```python
from build123d import *

# Parameters (mm, degrees)
BOSS_EXTRUDE1_DEPTH = 2.54
SKETCH2_R           = 2.032
CUT_EXTRUDE1_DEPTH  = 61.316926471


with BuildPart() as part:
    # Sketch1 → Boss-Extrude1 (new body)
    with BuildSketch(Plane.XY):
        with BuildLine():
            Line((-18.135713172, 23.369697581), (-2.946569758, 22.862546371))
            ThreePointArc((-2.946569758, 22.862546371), (1.365281203, 25.533694473), (0.557997895, 30.541227253))
            ThreePointArc((0.557997895, 30.541227253), (-21.942363625, 40.125896641), (-44.092394737, 29.757276792))
            ThreePointArc((-44.092394737, 29.757276792), (-43.193963557, 24.360517848), (-38.053791843, 26.234236193))
            ThreePointArc((-38.053791843, 26.234236193), (-37.941623484, 26.499357867), (-37.800175961, 26.750084494))
            ThreePointArc((-37.800175961, 26.750084494), (-33.769573387, 30.919616017), (-28.44204105, 33.2105))
            ThreePointArc((-28.44204105, 33.2105), (-21.549726751, 32.845355593), (-17.268032218, 27.432))
            Line((-17.268032218, 27.432), (-21.082, 26.416))
            ThreePointArc((-21.082, 26.416), (-20.2249274, 24.29700469), (-18.135713172, 23.369697581))
        make_face()
    extrude(amount=BOSS_EXTRUDE1_DEPTH)

    # Sketch2 → Cut-Extrude1 (cut, through all)
    with BuildSketch(Plane.XY.offset(2.54)):
        with Locations((-2.794, 27.432)):
            Circle(SKETCH2_R)
    extrude(amount=-CUT_EXTRUDE1_DEPTH, mode=Mode.SUBTRACT)


solid = part.part
```
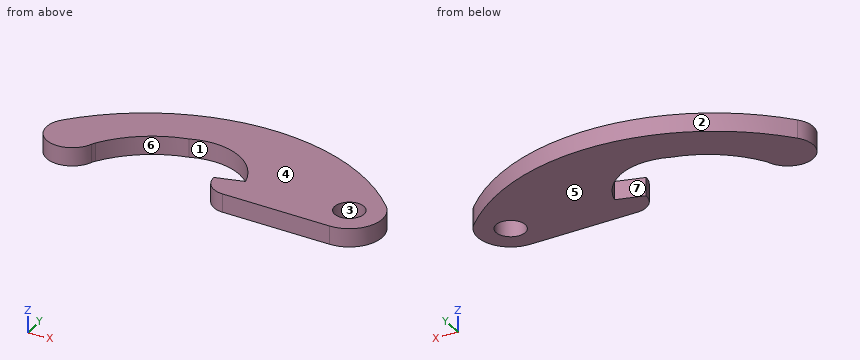
Geometry: final body of the model. Coordinates: model frame, mm. Face numbers are marked on the shaded views. A direction names the side the tool comes from. Give positions to 0.01 mm unless a question says otherwise; leave off trailing zeros. Loops run counter-clockwise (first coordinate to the right, second up) from the corner with the lowest first, then second, coordinate; pieces in that order, holes last. Notation, with made-up numbers: (59.25, 89.25) -> (63.25, 89.25) arc R10 ccw to (63.25, 99.25) -> close; hole circle Ø3 at (87, 64). An arc over 180 degrees is marked (long way). Use one line per item in the form item = value.
Item 1: Section query C-C on x = -26. Output: boundary loops of the cut face in (y, z), and give its area (3 significant figures).
A:
outline = (33.76, 0) -> (39.78, 0) -> (39.78, 2.54) -> (33.76, 2.54) -> close
area = 15.3 mm^2
Item 2: Draft query along X for the marked faces 1, 2, 3 and 4. Return one class per face: pulls with the +X half, pulls with the -X half, needs draft (parallel to the pull), parting line crosses it, or undercut.
A:
face_1 = undercut
face_2 = parting line crosses it
face_3 = undercut
face_4 = needs draft
Item 3: Section query A-A on z = 1.2. Output: boundary loops of the cut face in (x, y), and give its area (3 significant figures).
A:
outline = (-44.09, 29.76) arc R3.56 ccw (long way) to (-38.05, 26.23) arc R2.54 cw to (-37.8, 26.75) arc R14.73 cw to (-28.44, 33.21) arc R8.38 cw to (-17.27, 27.43) -> (-21.08, 26.42) arc R3.05 ccw to (-18.14, 23.37) -> (-2.95, 22.86) arc R4.57 ccw to (0.56, 30.54) arc R29.97 ccw to start; hole circle Ø4.06 at (-2.79, 27.43)
area = 442 mm^2
Item 4: Section query B-B on y = 28.5. Output: boundary loops of the cut face in (x, z), and give its area (3 significant figures).
A:
outline = (-44.79, 0) -> (-36.48, 0) -> (-36.48, 2.54) -> (-44.79, 2.54) -> close; (-17.61, 0) -> (-4.52, 0) -> (-4.52, 2.54) -> (-17.61, 2.54) -> close; (-1.07, 0) -> (1.65, 0) -> (1.65, 2.54) -> (-1.07, 2.54) -> close
area = 61.3 mm^2
Item 5: Section query D-D on y = 38.5. Output: boundary loops of the cut face in (x, z).
A:
outline = (-31.17, 0) -> (-11.67, 0) -> (-11.67, 2.54) -> (-31.17, 2.54) -> close
Item 6: Access query for the marked faces 5, 6 and 7. Directions: +Z, -Z, +X, -X, +Y, -Y. A direction counts if a zero-diameter tool reaches every point of the face in a straight line with its end or side. Return the directions, or none.
A:
face_5 = -Z, +X, -X, +Y, -Y
face_6 = +Z, -Z, -Y
face_7 = +Z, -Z
Item 7: Line query: probe 1 along X at (y, z) = (28, 0.6) (3 decimals); probe 2 along X at (y, z) = (26, 0.9); probe 3 along X at (y, z) = (32, 2.1). Output: solid intervals per line, ascending.
A:
probe_1 = -44.912 to -36.903, -17.431 to -4.745, -0.843 to 1.743
probe_2 = -44.66 to -38.15, -21.05 to -4.24, -1.35 to 1.55
probe_3 = -41.94 to -31.93, -20.23 to -0.89
